Check sheet for the modelled part. Datum: model origin and axes. Units: mm. Face numbers are marked on the shaded views. A direction names the side the tool comes from. Coordinates: 2 decimals unless noted, no trailing zeros. Loops run counter-clockwise (first coordinate to the right, second up) from the corner with the lowest first, then second, coordinate; pieces in that order, holes last. Notation, with made-up numbers: M -3,54.25 L 51,54.25 A24 cw 51,72.25 Z; hole C -12.5,59 d2. An arc over 180 degrees is marked long. Write each question's results on one line, items separated by ' | '. Start each with the question number.
from build123d import *

# Parameters (mm, degrees)
SKETCH1_R           = 2.5
SKETCH1_R_2         = 1.4
BOSS_EXTRUDE1_DEPTH = 7
BOSS_EXTRUDE2_REACH = 62.11
SKETCH2_W           = 0.9
SKETCH2_H           = 6.1
CUT_EXTRUDE1_REACH  = 62.11
SKETCH3_R           = 2.5


with BuildPart() as part:
    # Sketch1 → Boss-Extrude1 (new body)
    with BuildSketch(Plane.XY):
        with BuildLine():
            Line((3, 0), (12, 0))
            ThreePointArc((12, 0), (14.121320344, 0.878679656), (15, 3))
            Line((15, 3), (15, 16.267949192))
            Line((15, 16.267949192), (22.350852961, 29))
            Line((22.350852961, 29), (32.5, 29))
            ThreePointArc((32.5, 29), (34.621320344, 29.878679656), (35.5, 32))
            Line((35.5, 32), (35.5, 45))
            ThreePointArc((35.5, 45), (34.621320344, 47.121320344), (32.5, 48))
            Line((32.5, 48), (17.732050808, 48))
            ThreePointArc((17.732050808, 48), (16.232050808, 47.598076211), (15.133974596, 46.5))
            Line((15.133974596, 46.5), (0.401923789, 20.983339502))
            ThreePointArc((0.401923789, 20.983339502), (0.102222521, 20.259796637), (0, 19.483339502))
            Line((0, 19.483339502), (0, 3))
            ThreePointArc((0, 3), (0.878679656, 0.878679656), (3, 0))
        make_face()
        with Locations((25, 39)):
            Circle(SKETCH1_R, mode=Mode.SUBTRACT)
        with Locations((7.5, 5.4)):
            Circle(SKETCH1_R_2, mode=Mode.SUBTRACT)
        with Locations((7.5, 15)):
            Circle(SKETCH1_R_2, mode=Mode.SUBTRACT)
    extrude(amount=BOSS_EXTRUDE1_DEPTH)

    # Boss-Extrude2: up to this plane
    boss_extrude2_end = Plane(origin=(15.133974596, 46.5, 7), z_dir=(0.86602540378444, -0.4999999999999976, 0))
    # Sketch2 → Boss-Extrude2 (add, up to the surface)
    with BuildSketch(Plane(origin=(35.5, 0, 0), x_dir=(0, 0, -1), z_dir=(1, 0, 0)), mode=Mode.PRIVATE) as boss_extrude2_sk1:
        with Locations((0.45, 39)):
            Rectangle(SKETCH2_W, SKETCH2_H)
    boss_extrude2_tool1 = split(extrude(boss_extrude2_sk1.sketch, amount=-BOSS_EXTRUDE2_REACH, mode=Mode.PRIVATE), bisect_by=boss_extrude2_end, keep=Keep.BOTH, mode=Mode.PRIVATE)
    add(boss_extrude2_tool1.solids().sort_by_distance((35.5, 39, -0.45))[0])

    # Sketch3 → Cut-Extrude1 (cut, up to next)
    with BuildSketch(Plane.XY, mode=Mode.PRIVATE) as cut_extrude1_sk1:
        with Locations(Location((25, 39, 0), (0, 0, 270))):
            Circle(SKETCH3_R)
    cut_extrude1_tool1 = extrude(cut_extrude1_sk1.sketch, amount=-CUT_EXTRUDE1_REACH, mode=Mode.PRIVATE) & part.part
    add(cut_extrude1_tool1.solids().sort_by_distance((25, 39, 0))[0], mode=Mode.SUBTRACT)


solid = part.part
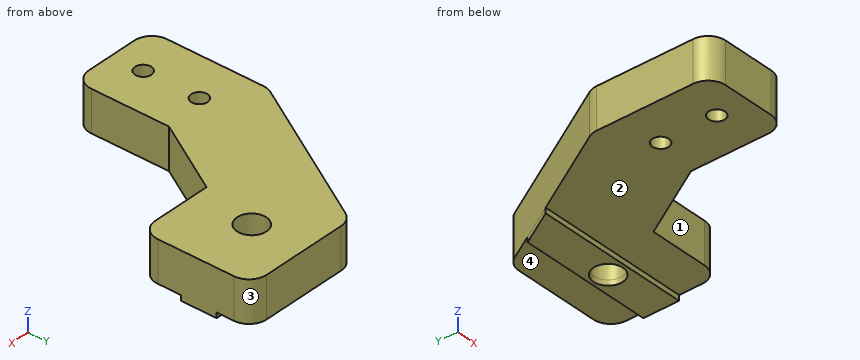
1) Section check A-A (x = 25). Enter the section's corners in (y, z).
2) Gauge pin test, flat ends, axial feed: P1, Ø0.7, axis at x = 20.5, z = -0.5, coming from the +Y side; P2, Ø3, axis at x = 25, y = 39, coming from the +Z side; P3, Ø3, axis at x = 30, y = 46, coming from the -Z side; P4, Ø3.5, axis at x = 28, z = 4.5, coming from the -Y side. Record the tip position at first contact, or that the pin passes through.
3) Section check D-D (x = 30). Enter the section's corners in (y, z), then the cut area to 3 significant figures.
4) Thickness scan on probe 1 along Y at (x, z) = (25, 5); probe 2 along X at (y, z) = (8.5, 6.5); probe 3 along Z at (x, y) = (14.5, 14). Record the ranges inside material, lowest first.
5) Section check C-C (z = 6.5). Enter the section's corners in (x, y), then the cut area to 3 significant figures.
6) Set-up check for the marked faces 1, 2, 3 and 4: record each of +Z, -Z, +X, -X, +Y, -Y from which the full face is reachable in a straight line by a thin tool's end or side.
7) Section check B-B (y = 5.4). Enter the section's corners in (x, z), then the cut area to 3 significant figures.
Return value:
1) outline: M 29,0 L 35.95,0 L 35.95,-0.9 L 36.5,-0.9 L 36.5,7 L 29,7 Z; M 41.5,-0.9 L 42.05,-0.9 L 42.05,0 L 48,0 L 48,7 L 41.5,7 Z
2) P1: stops at y = 42.05 | P2: passes through | P3: stops at z = 0 | P4: stops at y = 29
3) outline: M 29,0 L 35.95,0 L 35.95,-0.9 L 42.05,-0.9 L 42.05,0 L 48,0 L 48,7 L 29,7 Z | area: 138 mm2
4) probe 1: y = 29 to 36.5, 41.5 to 48 | probe 2: x = 0 to 15 | probe 3: z = 0 to 7
5) outline: M 0,3 A3 ccw 3,0 L 12,0 A3 ccw 15,3 L 15,16.27 L 22.35,29 L 32.5,29 A3 ccw 35.5,32 L 35.5,45 A3 ccw 32.5,48 L 17.73,48 A3 ccw 15.13,46.5 L 0.4,20.98 A3 ccw 0,19.48 Z; hole C 7.5,5.4 d2.8; hole C 7.5,15 d2.8; hole C 25,39 d5 | area: 894 mm2
6) face 1: +Z, -Z, +X, -Y | face 2: -Z, +X, -X, -Y | face 3: +Z, -Z, +X, +Y | face 4: -Z, +X, -X, +Y
7) outline: M 0,0 L 6.1,0 L 6.1,7 L 0,7 Z; M 8.9,0 L 15,0 L 15,7 L 8.9,7 Z | area: 85.4 mm2
